For this review, take the finished solid that the model builds, in its own axes (mm). Face numbers are marked on the shaded views. Round coordinates to 2 decimals unless told otherwise and drop trailing zeros. Loops run counter-clockwise (first coordinate to the right, second up) from the corner with the lowest first, then second, coordinate; pieces in that order, holes last. Notation, with made-up numbers: (-12, -30) -> (20, -30) arc R16 cw to (20, -17) -> close; hole circle Ø9 at (23.25, 48.5). An arc over 180 degrees is marked (long way). One line per question, with ' | ' between items. Start each with the question number.
1. Draft analysis for pull direction X (two halves, no side actions). For the marked faces 1 and 2, state which applies: pulls with the +X half, pulls with the -X half, needs draft (parallel to the pull), parting line crosses it, or undercut.
2. For pin 1 Ø2 at (y, z) = (0, -10) entering from +X; pin 2 Ø5 at (x, z) = (-23.75, 0) entering from +Y; pin 3 Ø16.5 at (x, z) = (12, 11.5) entering from -Y, all flat-tipped, find the tip position at first contact; note any pin that passes through.
3. Wall thickness on line 1 along Z through (x, y) = (0, 1.5); line 2 along Y through (x, z) = (-0.5, -17); line 3 along X through (y, z) = (0.5, -23.75): over which ranges is each line inside the solid? List them lowest first.
4. Consider section B-B (x = -23.75). Write out the cut boundary in (y, z), and give its area (3 significant figures).
5. Consider section C-C (y = 1). Count the separate pieces of the cut face and the enclosed holes in it, and give its area (3 significant figures).
6. Consider section A-A (z = 23.75). Write out the cut boundary in (x, y), and give its area (3 significant figures).
Autodesk Inventor part; units mm, degrees
ref_plane "YZ Plane" through (0, 0, 0) normal (1, 0, 0) x (0, 1, 0)
ref_plane "XZ Plane" through (0, 0, 0) normal (0, 1, 0) x (-1, 0, 0)
ref_plane "XY Plane" through (0, 0, 0) normal (0, 0, 1) x (1, 0, 0)
sketch "Boceto1" plane through (0, 0, 0) normal (0, 1, 0) x (-1, 0, 0)
  circle A0 centre (0, 0) radius 27.5
  dimension "d0" = 55
extrude "Extrusión1" add sketch "Boceto1" along normal blind 2
sketch "Boceto6" plane through (0, 2, 0) normal (0, 1, 0) x (1, 0, 0)
  circle A0 centre (0, 0) radius 9.6625
  circle A1 centre (-8.777, -8.777) radius 2.75
  circle A2 centre (0, 0) radius 7.1625
  circle A3 centre (8.4584, 0) radius 1
  circle A4 centre (0, -8.3447) radius 1
  circle A5 centre (0, 8.3727) radius 1
  circle A6 centre (-8.3635, 0) radius 1
  circle A7 centre (5.9357, -5.7822) radius 1
  circle A8 centre (-6.027, 5.9234) radius 1
  circle A9 centre (5.6693, 6.1791) radius 1
  circle A10 centre (-5.9197, -5.9092) radius 1
  dimension "d32" = 14.325
  dimension "d33" = 2
  dimension "d34" = 2
  dimension "d35" = 2
  dimension "d36" = 2
  dimension "d37" = 2
  dimension "d38" = 2
  dimension "d39" = 2
  dimension "d40" = 2
extrude "Extrusión3" cut sketch "Boceto6" against normal blind 50 contours A3 | A4 | A5 | A6 | A7 | A8 | A9 | A10
sketch "Boceto7" plane through (0, 0, 0) normal (0, 0, 1) x (1, 0, 0)
  line L0 (0, 0) -> (-7.1625, 0)
  line L1 (-11.527, 0) -> (-11.527, 2)
  line L2 (0, 0) -> (0, -5)
  line L3 (0, -5) -> (-7.1625, 0)
  dimension "d43" = 7.1625
  dimension "d44" = 5
revolve "Revolución2" add sketch "Boceto7" angle 360 about axis through (0, 0, 0) along (0, -1, 0)
sketch "Boceto8" plane through (0, 2, 0) normal (0, 1, 0) x (1, 0, 0)
  circle A0 centre (0, 0) radius 7.1625
  line L0 (0, 0) -> (0, 23.75)
  line L1 (0, 0) -> (23.75, 0)
  line L2 (0, 0) -> (0, -23.75)
  line L3 (0, 0) -> (-23.75, 0)
  circle A1 centre (-23.75, 0) radius 2.75
  circle A2 centre (0, 23.75) radius 2.75
  circle A3 centre (23.75, 0) radius 2.75
  circle A4 centre (0, -23.75) radius 2.75
  point P0 (0, 0)
  dimension "d57" = 23.75
  dimension "d58" = 23.75
  dimension "d59" = 23.75
  dimension "d60" = 23.75
  dimension "d61" = 5.5
  dimension "d62" = 5.5
  dimension "d63" = 5.5
  dimension "d64" = 5.5
extrude "Extrusión4" cut sketch "Boceto8" against normal blind 2 contours A4 | A1 | A2 | A3
sketch "Boceto10" plane through (0, 2, 0) normal (0, 1, 0) x (1, 0, 0)
  point P0 (0, 0)
properties part number "placa para pellet"
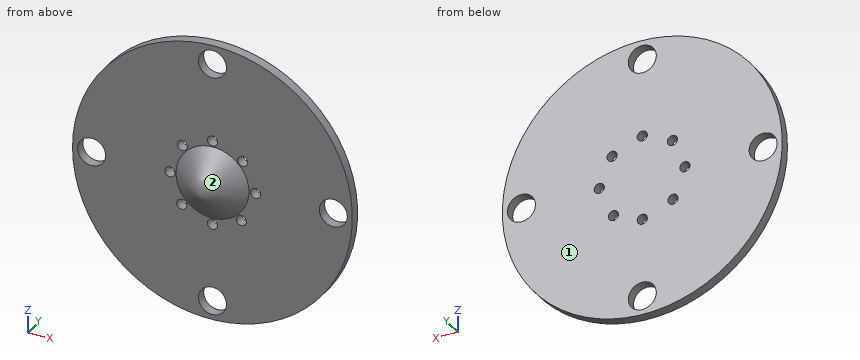
Answer block:
1) face 1: needs draft | face 2: parting line crosses it
2) pin 1: stops at x = 25.99 | pin 2: passes through | pin 3: stops at y = 0
3) line 1: z = -27.5 to -26.5, -21 to -9.37, -7.37 to 7.34, 9.34 to 21, 26.5 to 27.5 | line 2: y = 0 to 2 | line 3: x = -13.86 to -2.75, 2.75 to 13.86
4) outline: (0, -13.86) -> (2, -13.86) -> (2, -2.75) -> (0, -2.75) -> close; (0, 2.75) -> (2, 2.75) -> (2, 13.86) -> (0, 13.86) -> close | area: 44.5 mm2
5) separate pieces: 1 | enclosed holes: 12 | area: 2,260 mm2
6) outline: (-13.86, 0) -> (-2.75, 0) -> (-2.75, 2) -> (-13.86, 2) -> close; (2.75, 0) -> (13.86, 0) -> (13.86, 2) -> (2.75, 2) -> close | area: 44.5 mm2
